Autodesk Fusion 360 part; units mm, degrees
cylinder "CylinderPrimitive1" add diameter 50.8 height 3.175 placed x (1, 0, 0) y (0, 1, 0) z (0, 0, 1) at (0, 0, 0) in component "Sandblaster Cabinet pegs"
cylinder "CylinderPrimitive2" add diameter 19.05 height 3.175 placed x (1, 0, 0) y (0, 1, 0) z (0, 0, 1) at (0, 0, 3.175) in component "Sandblaster Cabinet pegs"
hole "Hole1" at (0, 0, 6.35) direction (0, 0, -1) diameter 3.429 end through all countersink diameter 4.7625 countersink angle 82 in component "Sandblaster Cabinet pegs"
chamfer "Chamfer1" distance 0.7937 angle 45 1 edges at (-23.6811, -9.185, 3.175) in component "Sandblaster Cabinet pegs"
component "Sandblaster Cabinet pegs" placed x (1, 0, 0) y (0, 1, 0) z (0, 0, 1) at (0, 0, 0)
equation "d12 = ( 1 / 32 ) * 1 in"
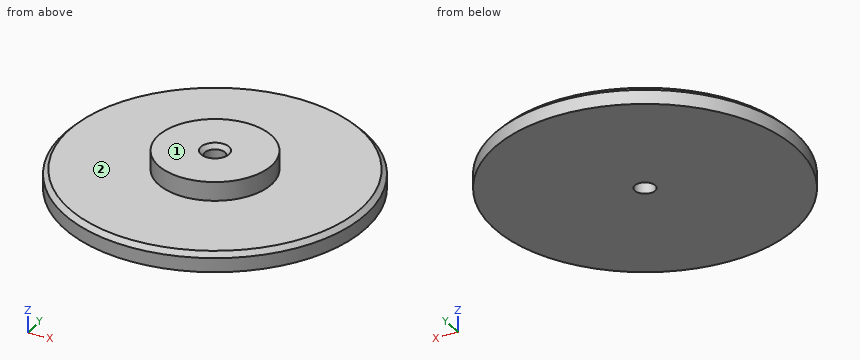
Verification items for the finished model (mm, model axes). Face numbers are marked on the shaded views. A direction names the side the tool comes from. Round coordinates to 2 decimals unless told otherwise and drop trailing zeros. Loops run counter-clockwise (first coordinate to the right, second up) from the corner with the lowest first, then second, coordinate; pieces in that order, holes last. Notation, with made-up numbers: (54, 16) - (93, 16) arc R10 ccw to (93, 20) - close; hole circle Ø6 at (78, 75.5). An arc over 180 degrees is marked (long way). Answer in a Markdown table with one row per item. Add a question column.
Q1. Section check C-C on z = 1.5. Enter the section's corners in (x, y), plus the area to 3 significant figures.
Q2. Tool access check on the marked faces 1 and 2. Record the directions out of +Z, -Z, +X, -X, +Y, -Y that give a thin tool (end or side, any length) a straight path to the whole face; none if there is none.
Q3. Gauge pin test, flat ends, axial feed: pin 1 (8 mm diameter, centred on x = 16, y = 2, fed in from +Z) (3 decimals); pin 2 (1 mm diameter, centred on y = -19.5, z = 1, fed in from +X); pin 3 (2 mm diameter, centred on y = 2, z = 4, fed in from -X). Record the tip position at first contact, or that the pin passes through.
Q4. Material ranges on line 1 (Y direction, x = 0, z = 1.3); line 2 (Y direction, x = 0, z = 3.45) (1 decimal); line 3 (Z direction, x = -17, y = -16.5) (3 decimals), recorded low to high.
Found:
| question | item | result |
|---|---|---|
| 1 | outline | circle Ø50.8 at (0, 0); hole circle Ø3.43 at (0, 0) |
| 1 | area | 2,020 mm² |
| 2 | face 1 | +Z, +X, -X, +Y, -Y |
| 2 | face 2 | +Z |
| 3 | pin 1 | stops at z = 3.175 |
| 3 | pin 2 | stops at x = 16.86 |
| 3 | pin 3 | stops at x = -24.7 |
| 4 | line 1 | y = -25.4 to -1.71, 1.71 to 25.4 |
| 4 | line 2 | y = -9.5 to -1.7, 1.7 to 9.5 |
| 4 | line 3 | z = 0 to 3.175 |
